Source: three-view drawing plus pictorial views. Frame: mm from the lowest corner of the part. A direction names the side the tool comes from. Round coordinates to 2 decimals unless told otherwise and drop trailing zeros. Order: outer loops, then holes, each group sorted by start corner. A loop starts at its lowest first (then second) coordinate and runs counter-clockwise, first axis right, second up. Notation, with made-up numbers: (47.25, 47) -> (105.25, 47) arc R15 ccw to (105.25, 53) -> close; hole circle Ø5 at (49, -35). An arc over 180 degrees is marked (long way). Use a Markdown table: item, result.
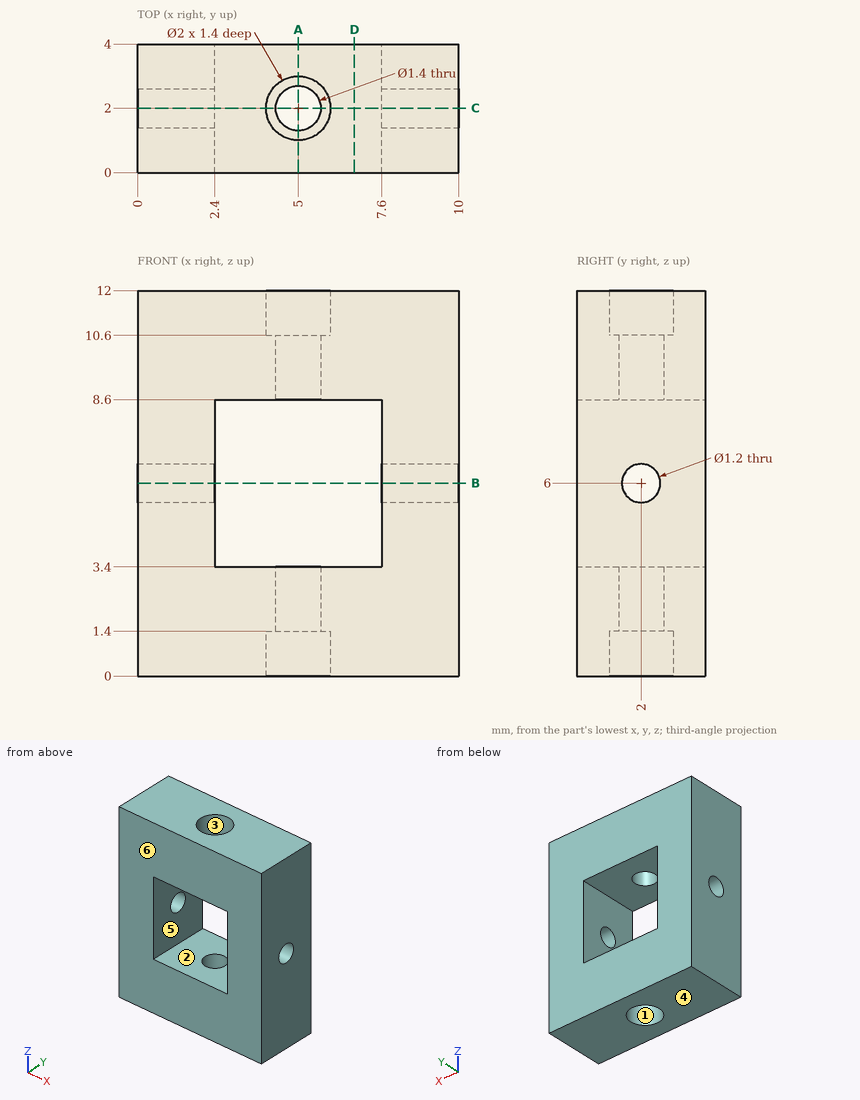
1) Cut plane C-C on y = 2. Count the separate pieces of the cut face and the enclosed holes in it, and give its area (3 significant figures).
Results found:
| item | result |
|---|---|
| separate pieces | 4 |
| enclosed holes | 0 |
| area | 76.0 mm² |
2) Pin query (flat end, axial travel): pin 1 Ø1.8 at (x, y) = (5, 2) entering from +Z; pin 2 Ø3 at (x, z) = (4.5, 6) entering from +Y. Return the tip coordinate at first contact, or that it passes through.
Results found:
| item | result |
|---|---|
| pin 1 | stops at z = 10.6 |
| pin 2 | passes through |
3) Pull-direction query (Z, two-part tool) for the marked faces 4, 5 and 6; classes: +Z half, -Z half, draft (parallel to the pull), parting line (faces both ways), or undercut.
Results found:
| item | result |
|---|---|
| face 4 | -Z half |
| face 5 | undercut |
| face 6 | draft |
4) Cut plane D-D on x = 6.75. Return loops of the section in (y, z).
Results found:
| item | result |
|---|---|
| outline | (0, 0) -> (4, 0) -> (4, 3.4) -> (0, 3.4) -> close; (0, 8.6) -> (4, 8.6) -> (4, 12) -> (0, 12) -> close |
5) Line query: L1, parallel to Z at x = 6, y = 2.95; L2, parallel to X at y = 1.7, z = 4; L3, parallel to Y at x = 5, z = 2. Output: solid intervals per line, ascending. Write a range as [from, to].
Results found:
| item | result |
|---|---|
| L1 | z = [0, 3.4], [8.6, 12] |
| L2 | x = [0, 2.4], [7.6, 10] |
| L3 | y = [0, 1.3], [2.7, 4] |
6) Cut plane B-B on z = 6. Return loops of the section in (x, y).
Results found:
| item | result |
|---|---|
| outline | (0, 0) -> (2.4, 0) -> (2.4, 1.4) -> (0, 1.4) -> close; (0, 2.6) -> (2.4, 2.6) -> (2.4, 4) -> (0, 4) -> close; (7.6, 0) -> (10, 0) -> (10, 1.4) -> (7.6, 1.4) -> close; (7.6, 2.6) -> (10, 2.6) -> (10, 4) -> (7.6, 4) -> close |
7) Set-up query: the marked faces 1, 2 and 3. Return all of +Z, -Z, +X, -X, +Y, -Y with unobstructed straight access to the full face (end or side cutting, diameter ignored); none if empty.
Results found:
| item | result |
|---|---|
| face 1 | -Z |
| face 2 | +Y, -Y |
| face 3 | +Z |
8) Cut plane A-A on x = 5. Return loops of the section in (y, z), and give its area (3 significant figures).
Results found:
| item | result |
|---|---|
| outline | (0, 0) -> (1, 0) -> (1, 1.4) -> (1.3, 1.4) -> (1.3, 3.4) -> (0, 3.4) -> close; (0, 8.6) -> (1.3, 8.6) -> (1.3, 10.6) -> (1, 10.6) -> (1, 12) -> (0, 12) -> close; (2.7, 1.4) -> (3, 1.4) -> (3, 0) -> (4, 0) -> (4, 3.4) -> (2.7, 3.4) -> close; (2.7, 8.6) -> (4, 8.6) -> (4, 12) -> (3, 12) -> (3, 10.6) -> (2.7, 10.6) -> close |
| area | 16.0 mm² |
